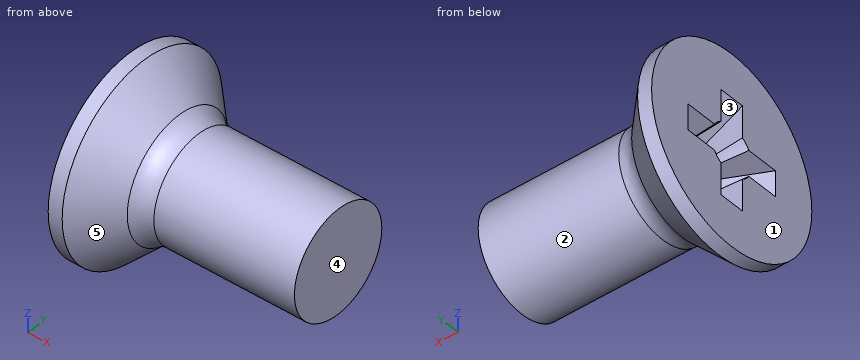
```python
from build123d import *

# Parameters (mm, degrees)
FILLET1_R    = 0.8
SKETCH3_W    = 0.74
SKETCH3_H    = 3
SKETCH4_W    = 0.74
SKETCH4_H    = 0.995702004
RECPAT_COUNT = 2
RECPAT_ANGLE = 90


with BuildPart() as part:
    # BodySke → Base-Revolve (revolve)
    with BuildSketch(Plane.XY):
        Polygon((0, 0), (0, 2.75), (0.4, 2.75), (1.65, 1.5), (6, 1.5), (6, 0), align=None)
    revolve(axis=Axis((-6.35, 0, 0), (1, 0, 0)))

    # Fillet1
    fillet1_edges = [part.edges().sort_by_distance(p)[0] for p in [
        (1.65, -1.5, 0),
    ]]
    fillet(fillet1_edges, radius=FILLET1_R)

    # Sketch3 → Recess section 0
    with BuildSketch(Plane.ZY):
        Rectangle(SKETCH3_W, SKETCH3_H)
    # Sketch4 → Recess section 1
    with BuildSketch(Plane.ZY.offset(-2.01)):
        Rectangle(SKETCH4_W, SKETCH4_H)
    recess = loft(mode=Mode.SUBTRACT)

    # RecPat: Recess ×2 about axis
    recpat_axis = Axis((0, 0, 0), (1, 0, 0))
    for i in range(1, RECPAT_COUNT):
        add(recess.rotate(recpat_axis, i * RECPAT_ANGLE / (RECPAT_COUNT - 1)), mode=Mode.SUBTRACT)

    # RecCorSke → RecessCore (revolve, cut)
    with BuildSketch(Plane.XY):
        Polygon((0, 0), (0, 0.696552892), (2.01, 0.556), (2.190655351, 0), align=None)
    revolve(axis=Axis((-3.175, 0, 0), (1, 0, 0)), mode=Mode.SUBTRACT)


solid = part.part
```
CAD build for the part. Positions are in the model's coordinates, mm. Face numbers are marked on the shaded views. A direction names the side the tool comes from. Give positions to 0.01 mm unless a question says otherwise; leave off trailing zeros. Order: outer loops, then holes, each group sorted by start corner. A loop starts at its lowest first (then second) coordinate and runs counter-clockwise, first axis right, second up. Notation, with made-up numbers: M 77.5,66.5 L 115.5,66.5 A23 cw 115.5,75.5 Z; hole C 4.25,18 d11. An arc over 180 degrees is marked long. Put each result on its own line as item: value. Start each with the question number.
(1) Saw through at A-A, the plane x = 4. Write the cut outline in (y, z), then the cut area to 3 significant figures.
(2) Flat gauge pins, fed straight in: pin 1 Ø3 at (x, z) = (5.5, -1.5) entering from -Y; pin 2 Ø1 at (x, y) = (1.5, -0.5) entering from +Z; pin 3 Ø1 at (x, y) = (4.5, -1) entering from +Z. Where does each tip first touch, or does it go through?
(3) Mould opens along Z. For the marked faces 3, 4 and 5 say: +Z half, -Z half, draft (parallel to the pull), parting line (faces both ways), or undercut.
(4) Drill centre lines: line 1 along Y through (x, z) = (1, -0.8); line 2 along Y through (x, z) = (0.5, -1.15); line 3 along Y through (x, z) = (4.5, 0.05). Where is each one in solid material? Low to high.
(5) Which spindle directions (+Z, -Z, +X, -X, +Y, -Y) get a long thin tool onto all of the face, cutting with end or side? Do the marked faces 1 and 2. Say none if no direction does.
Check result:
1. outline: C 0,0 d3
1. area: 7.07 mm2
2. pin 1: stops at y = -1.5
2. pin 2: stops at z = 2.1
2. pin 3: stops at z = 1.41
3. face 3: undercut
3. face 4: draft
3. face 5: parting line
4. line 1: y = -2 to -0.37, 0.37 to 2
4. line 2: y = -2.39 to -0.37, 0.37 to 2.39
4. line 3: y = -1.5 to 1.5
5. face 1: +Z, -Z, -X, +Y, -Y
5. face 2: +X
